```python
from build123d import *

# Parameters (mm, degrees)
SKETCH_1_R          = 37
EXTRUDE_1_DEPTH     = 7
SKETCH_2_R          = 35
EXTRUDE_2_DEPTH     = 13.5
SKETCH_3_R          = 27
EXTRUDE_3_DEPTH     = 12.5
SKETCH_4_R          = 18
EXTRUDE_4_DEPTH     = 7.5
EXTRUDE_START       = 5.5
SKETCH_5_R          = 18
EXTRUDE_5_DEPTH     = 5.5
SKETCH_6_R          = 10
EXTRUDE_6_DEPTH     = 6.5
SKETCH_7_R          = 7
CUT_EXTRUDE_1_DEPTH = 52.5
SKETCH_8_R          = 1.75
CUT_EXTRUDE_2_DEPTH = 20.5
SKETCH_9_R          = 1.5
CUT_EXTRUDE_3_DEPTH = 10


with BuildPart() as part:
    # Эскиз1 → Бобышка-Вытянуть1 (new body)
    with BuildSketch(Plane.XY):
        Circle(SKETCH_1_R)
    extrude(amount=EXTRUDE_1_DEPTH)

    # Эскиз2 → Бобышка-Вытянуть2 (add)
    with BuildSketch(Plane.XY.offset(7)):
        Circle(SKETCH_2_R)
    extrude(amount=EXTRUDE_2_DEPTH)

    # Эскиз3 → Бобышка-Вытянуть3 (add)
    with BuildSketch(Plane.XY.offset(20.5)):
        Circle(SKETCH_3_R)
    extrude(amount=EXTRUDE_3_DEPTH)

    # Эскиз4 → Бобышка-Вытянуть4 (add)
    with BuildSketch(Plane.XY.offset(33)):
        Circle(SKETCH_4_R)
    extrude(amount=EXTRUDE_4_DEPTH)

    # Эскиз5 → Бобышка-Вытянуть5 (add)
    with BuildSketch(Plane(origin=(0, 0, 0), x_dir=(-1, 0, 0), z_dir=(0, 0, -1)).offset(EXTRUDE_START)):
        with Locations(Location((0, 0, 0), (0, 0, 180))):
            Circle(SKETCH_5_R)
    extrude(amount=-EXTRUDE_5_DEPTH)

    # Эскиз6 → Бобышка-Вытянуть6 (add)
    with BuildSketch(Plane(origin=(0, 0, -5.5), x_dir=(-1, 0, 0), z_dir=(0, 0, -1))):
        with Locations(Location((0, 0, 0), (0, 0, 180))):
            Circle(SKETCH_6_R)
    extrude(amount=EXTRUDE_6_DEPTH)

    # Эскиз7 → Вырез-Вытянуть1 (cut)
    with BuildSketch(Plane(origin=(0, 0, -12), x_dir=(-1, 0, 0), z_dir=(0, 0, -1))):
        Circle(SKETCH_7_R)
    extrude(amount=-CUT_EXTRUDE_1_DEPTH, mode=Mode.SUBTRACT)

    # Эскиз8 → Вырез-Вытянуть2 (cut)
    with BuildSketch(Plane.XY.offset(20.5)):
        with Locations((0, 32)):
            Circle(SKETCH_8_R)
        with Locations((22.627416998, 22.627416998)):
            Circle(SKETCH_8_R)
        with Locations((32, 0)):
            Circle(SKETCH_8_R)
        with Locations((22.627416998, -22.627416998)):
            Circle(SKETCH_8_R)
        with Locations((0, -32)):
            Circle(SKETCH_8_R)
        with Locations((-22.627416998, -22.627416998)):
            Circle(SKETCH_8_R)
        with Locations((-32, 0)):
            Circle(SKETCH_8_R)
        with Locations((-22.627416998, 22.627416998)):
            Circle(SKETCH_8_R)
    extrude(amount=-CUT_EXTRUDE_2_DEPTH, mode=Mode.SUBTRACT)

    # Эскиз9 → Вырез-Вытянуть3 (cut)
    with BuildSketch(Plane.XY.offset(33)):
        with Locations((0, 22)):
            Circle(SKETCH_9_R)
        with Locations((11, 19.052558883)):
            Circle(SKETCH_9_R)
        with Locations((19.052558883, 11)):
            Circle(SKETCH_9_R)
        with Locations((22, 0)):
            Circle(SKETCH_9_R)
        with Locations((19.052558883, -11)):
            Circle(SKETCH_9_R)
        with Locations((11, -19.052558883)):
            Circle(SKETCH_9_R)
        with Locations((0, -22)):
            Circle(SKETCH_9_R)
        with Locations((-11, -19.052558883)):
            Circle(SKETCH_9_R)
        with Locations((-19.052558883, -11)):
            Circle(SKETCH_9_R)
        with Locations((-22, 0)):
            Circle(SKETCH_9_R)
        with Locations((-19.052558883, 11)):
            Circle(SKETCH_9_R)
        with Locations((-11, 19.052558883)):
            Circle(SKETCH_9_R)
    extrude(amount=-CUT_EXTRUDE_3_DEPTH, mode=Mode.SUBTRACT)


solid = part.part
```
Here's how the part is built. I have some questions about the finished solid (model axes, mm). A direction names the side the tool comes from. Give positions to 0.01 mm unless a question says otherwise; leave off trailing zeros. Write each loop counter-clockwise with the first axis right and the second up, starting at its lowest first coordinate (ties: lowest second). Pieces come first, ordered by that corner, then holes. Notation, with made-up numbers: (-4, 47.25) -> (3, 47.25) arc R24 ccw to (3, 85.25) -> close; hole circle Ø4 at (8.5, 21.25). An arc over 180 degrees is marked (long way). Use one line per item in the form item = value.
1) Suppose I cut it at B-B (z = 31). Give the number of separate pieces and of enclosed holes in the cut face, and give its area (3 significant figures).
Verdict:
separate_pieces = 1
enclosed_holes = 13
area = 2,050 mm2
2) I'm going to push flat-ended pins straight in: pin 1 (3.5 mm diameter, centred on x = -19.05, y = 11, fed in from -Z); pin 2 (2.5 mm diameter, centred on x = 10.5, y = 18.5, fed in from +Z); pin 3 (5.5 mm diameter, centred on x = -22.63, y = -22.63, fed in from +Z); pin 4 (8 mm diameter, centred on y = 0.5, z = 4, fed in from -X). Where does each tip first touch, or does it pass through?
Verdict:
pin_1 = 0
pin_2 = 33
pin_3 = 20.5
pin_4 = -37
3) We'd pull the mould along X, two halves only. Please class faces 1 (the face through (11, -19, 23)), 2 (the face through (-5.85, -26.36, 26.66)), 3 (the face through (-26, -8, 20.5)): +X half, -X half, draft (parallel to the pull), parting line (faces both ways), or undercut.
Verdict:
face_1 = undercut
face_2 = parting line
face_3 = draft
4) If I drill on L1, parallel to Y at x = 0, z = 27.5; L2, parallel to Y at x = 0, z = 9.75; L3, parallel to Y at x = -22, z = 4, over which ranges is the centre line in solid material (lowest first)? Write a range as [from, to].
Verdict:
L1 = [-27, -23.5], [-20.5, -7], [7, 20.5], [23.5, 27]
L2 = [-35, -33.75], [-30.25, -7], [7, 30.25], [33.75, 35]
L3 = [-29.75, -24.26], [-20.99, 20.99], [24.26, 29.75]
5) Suppose I cut it at C-C (y = -32). Please give me the cut outline in (x, z), and give its area (3 significant figures).
Verdict:
outline = (-18.57, 0) -> (-1.75, 0) -> (-1.75, 20.5) -> (-14.18, 20.5) -> (-14.18, 7) -> (-18.57, 7) -> close; (1.75, 0) -> (18.57, 0) -> (18.57, 7) -> (14.18, 7) -> (14.18, 20.5) -> (1.75, 20.5) -> close
area = 571 mm2
6) Suppose I cut it at D-D (z = 22). Please give me the cut outline in (x, y).
Verdict:
outline = circle Ø54 at (0, 0); hole circle Ø14 at (0, 0)
7) Suppose I cut it at A-A (x = -5.5). Please give me the cut outline in (y, z), and give its area (3 significant figures).
Verdict:
outline = (-36.59, 0) -> (-17.14, 0) -> (-17.14, -5.5) -> (-8.35, -5.5) -> (-8.35, -12) -> (-4.33, -12) -> (-4.33, 40.5) -> (-17.14, 40.5) -> (-17.14, 33) -> (-26.43, 33) -> (-26.43, 20.5) -> (-34.57, 20.5) -> (-34.57, 7) -> (-36.59, 7) -> close; (4.33, -12) -> (8.35, -12) -> (8.35, -5.5) -> (17.14, -5.5) -> (17.14, 0) -> (36.59, 0) -> (36.59, 7) -> (34.57, 7) -> (34.57, 20.5) -> (26.43, 20.5) -> (26.43, 33) -> (17.14, 33) -> (17.14, 40.5) -> (4.33, 40.5) -> close
area = 2,210 mm2
8) On a 3-axis mill with a long thin cutter (end or side, diameter ignored), from which of +Z, -Z, +X, -X, +Y, -Y can I reach the whole of each face in a straight line? I mean faces 4 (the face through (-28, -21, 14)), 5 (the face through (-33.75, 0.08, 10.39)), 6 (the face through (-10, 0, -9)). Say none if no direction works.
Verdict:
face_4 = +Z
face_5 = +Z, -Z
face_6 = -Z
